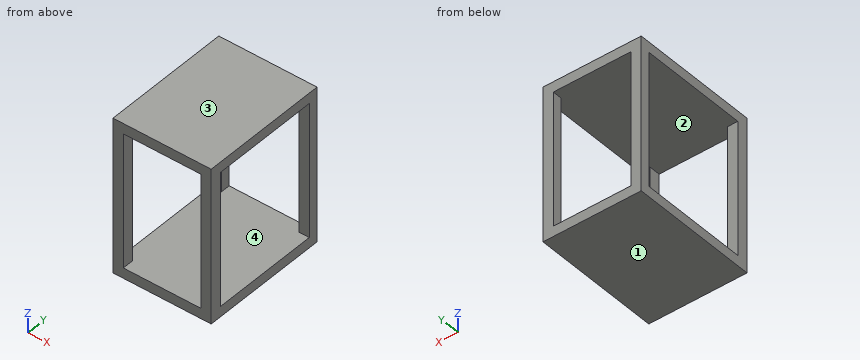
from build123d import *

# Parameters (mm, degrees)
F0_W     = 381
F0_H     = 50.8
F1_DEPTH = 635
F2_W     = 533.4
F2_H     = 660.4
F3_DEPTH = 482.601
F0_H_2   = 660.4
F4_DEPTH = 635.001


# Not quite as in the source:
# - a feature names something its author has since deleted; it is built from what else it names


with BuildPart() as f1:
    # F0 (on Front) → F1 (new body)
    with BuildSketch(Plane.XZ):
        with Locations((0, 355.6)):
            Rectangle(F0_W, F0_H)
        Polygon((241.3, 381), (190.5, 381), (190.5, 330.2), (190.5, -330.2), (190.5, -381), (241.3, -381), align=None)
        with Locations((0, -355.6)):
            Rectangle(F0_W, F0_H)
        Polygon((-190.5, 381), (-241.3, 381), (-241.3, -381), (-190.5, -381), (-190.5, -330.2), (-190.5, 330.2), align=None)
    extrude(amount=-F1_DEPTH)

    # F2 (on face) → F3 (cut, through all)
    with BuildSketch(Plane.YZ.offset(241.3)):
        with Locations((321.7956796288, 0)):
            Rectangle(F2_W, F2_H)
    extrude(amount=-F3_DEPTH, mode=Mode.SUBTRACT)

    # F0 (on Front) → F4 (cut, through all)
    with BuildSketch(Plane.XZ):
        Rectangle(F0_W, F0_H_2)
    extrude(amount=-F4_DEPTH, mode=Mode.SUBTRACT)


solid = f1.part
Can you work these out from the model? Positions are in its coordinate system, mm. Face numbers are marked on the shaded views. A direction names the side the tool comes from. Coordinates: 2 decimals unless noted, no trailing zeros. Order: outer loops, then holes, each group sorted by start corner. A loop starts at its lowest first (then second) coordinate and runs counter-clockwise, first axis right, second up. Notation, with made-up numbers: (34, 24.5) - (76, 24.5) arc R27 ccw to (76, 50.5) - close; hole circle Ø1 at (-5, -29). An arc over 180 degrees is marked (long way). Answer as a JSON object with one key per item and string values. Group by question number.
Q1. I need wall thicknesses on line 1 (Z direction, x = 174, y = 461). Which ranges of the line are inside material? Lowest first, please. Write a range as from..to.
Q2. On a 3-axis mill with a long thin cutter (end or side, diameter ignored), from which of +Z, -Z, +X, -X, +Y, -Y can I reach the whole of each face in a straight line? I mean the marked faces 3 and 4. Say none if no direction works.
Q3. Imagine slicing it at A-A (y = 524). Please give me the cut outline in (x, z).
Q4. Imagine slicing it at D-D (x = 209). Please give me the cut outline in (y, z).
Q5. We'd pull the mould along X, two halves only. Please class the marked faces 1 and 2: +X half, -X half, draft (parallel to the pull), parting line (faces both ways), or undercut.
Q6. Imagine slicing it at C-C (z = -2). Please give me the cut outline in (x, y).
Q7. Imagine slicing it at B-B (x = 112). Please give me the cut outline in (y, z).
Determined:
{
 "1": {"line 1": "z = -381..-330.2, 330.2..381"},
 "2": {"face 3": "+Z, +X, -X, +Y, -Y", "face 4": "none"},
 "3": {"outline": "(-241.3, -381) - (241.3, -381) - (241.3, -330.2) - (-241.3, -330.2) - close; (-241.3, 330.2) - (241.3, 330.2) - (241.3, 381) - (-241.3, 381) - close"},
 "4": {"outline": "(0, -381) - (635, -381) - (635, 381) - (0, 381) - close; hole (55.1, -330.2) - (588.5, -330.2) - (588.5, 330.2) - (55.1, 330.2) - close"},
 "5": {"face 1": "draft", "face 2": "undercut"},
 "6": {"outline": "(-241.3, 0) - (-190.5, 0) - (-190.5, 55.1) - (-241.3, 55.1) - close; (-241.3, 588.5) - (-190.5, 588.5) - (-190.5, 635) - (-241.3, 635) - close; (190.5, 0) - (241.3, 0) - (241.3, 55.1) - (190.5, 55.1) - close; (190.5, 588.5) - (241.3, 588.5) - (241.3, 635) - (190.5, 635) - close"},
 "7": {"outline": "(0, -381) - (635, -381) - (635, -330.2) - (0, -330.2) - close; (0, 330.2) - (635, 330.2) - (635, 381) - (0, 381) - close"}
}
